Could you check a few things on this model? Use its own coordinates, in mm. A direction names the side the tool comes from. Coordinates: 2 decimals unless noted, no trailing zeros. Loops run counter-clockwise (first coordinate to the right, second up) from the corner with the lowest first, then second, coordinate; pieces in that order, holes last. Notation, with made-up numbers: (-3.5, 87.5) -> (4.5, 87.5) arc R19 cw to (4.5, 112.5) -> close; hole circle Ø11 at (48.25, 52.5). An arc over 180 degrees is marked (long way). One line per question, with ' | ' between items. Start each with the question number.
(1) If we mould it in two halves opening along Y, with no side actions, what happens to faces 1 (the face through (-6.883, -30.995, 6.261)), 2 (the face through (-22.37, 0.95, 6.44)), 3 (the face through (7, -7, 25.4))? For each: pulls with the +Y half, pulls with the -Y half, needs draft (parallel to the pull), parting line crosses it, or undercut.
(2) Suppose I cut it at A-A (y = 0). Please give me the cut outline in (x, z) (3 decimals), plus the area to 3 significant figures.
(3) I'm going to push flat-ended pins straight in: pin 1 Ø8 at (y, z) = (4.5, 22) entering from +X; pin 2 Ø10 at (y, z) = (15.5, 7) entering from -X; pin 3 Ø6 at (x, z) = (16.5, 19.5) entering from +Y. Where does each tip first touch, or does it pass through?
(4) Suppose I cut it at C-C (x = -25.4). Please give me the cut outline in (y, z) (3 decimals), plus the area to 3 significant figures.
(5) If I drill on line 1 along Y through (x, z) = (0, 9.75) (3 decimals); line 2 along Y through (x, z) = (0, 18) (3 decimals); line 3 along Z through (x, y) = (8, -2.5), over which ranges is the centre line in solid material (lowest first)?
(6) Which directions (+Z, -Z, +X, -X, +Y, -Y) give clear straight access to the entire face, cutting with the end or side of a thin tool? Please do faces 4 (the face through (-0.41, 28.55, 6.44)), 5 (the face through (7, 15, 12.7)).
```python
from build123d import *

# Parameters (mm, degrees)
F0_R     = 31.75
F1_DEPTH = 12.7
F2_R     = 3.175
F3_DEPTH = 12.701
F2_R_2   = 15.875
F2_R_3   = 9.525
F4_DEPTH = 12.7


with BuildPart() as f1:
    # F0 (on Top) → F1 (new body)
    with BuildSketch(Plane.XY):
        Circle(F0_R)
    extrude(amount=F1_DEPTH)

    # F2 (on face) → F3 (cut, through all)
    with BuildSketch(Plane.XY.offset(12.7)):
        with Locations((-25.4, 0)):
            Circle(F2_R)
        with Locations((0, -25.4)):
            Circle(F2_R)
        with Locations((25.4, 0)):
            Circle(F2_R)
        with Locations((0, 25.4)):
            Circle(F2_R)
    extrude(amount=-F3_DEPTH, mode=Mode.SUBTRACT)

    # F2 (on face) → F4 (join)
    with BuildSketch(Plane.XY.offset(12.7)):
        Circle(F2_R_2)
        Circle(F2_R_3, mode=Mode.SUBTRACT)
    extrude(amount=F4_DEPTH)


solid = f1.part
```
Checks:
1) face 1: parting line crosses it | face 2: undercut | face 3: needs draft
2) outline: (-31.75, 0) -> (-28.575, 0) -> (-28.575, 12.7) -> (-31.75, 12.7) -> close; (-22.225, 0) -> (22.225, 0) -> (22.225, 12.7) -> (15.875, 12.7) -> (15.875, 25.4) -> (9.525, 25.4) -> (9.525, 12.7) -> (-9.525, 12.7) -> (-9.525, 25.4) -> (-15.875, 25.4) -> (-15.875, 12.7) -> (-22.225, 12.7) -> close; (28.575, 0) -> (31.75, 0) -> (31.75, 12.7) -> (28.575, 12.7) -> close | area: 806 mm^2
3) pin 1: stops at x = 15.87 | pin 2: stops at x = -29.96 | pin 3: stops at y = 8.35
4) outline: (-19.05, 0) -> (-3.175, 0) -> (-3.175, 12.7) -> (-19.05, 12.7) -> close; (3.175, 0) -> (19.05, 0) -> (19.05, 12.7) -> (3.175, 12.7) -> close | area: 403 mm^2
5) line 1: y = -31.75 to -28.575, -22.225 to 22.225, 28.575 to 31.75 | line 2: y = -15.875 to -9.525, 9.525 to 15.875 | line 3: z = 0 to 12.7
6) face 4: +Z, -Z | face 5: +Z
